Input: part model. Units: mm. Frame: model coordinates. Give positions to 0.01 mm unless a question says otherwise; leave off trailing zeros. Loops run counter-clockwise (first coordinate to the right, second up) from the corner with the lowest first, then second, coordinate; pieces in that order, holes last. Notation, with made-up numbers: (-23.75, -10.5) -> (-18.75, -10.5) arc R24 cw to (-18.75, 24.5) -> close; hole circle Ø6 at (15.5, -34.5). An arc over 180 degrees is marked (long way). Answer as a JSON object with one key per item and string values. Group by question number.
```python
from build123d import *

# Parameters (mm, degrees)
BASE_FLANGE1_DEPTH       = 2
SKETCH3_W                = 15
SKETCH3_H                = 15
TAB1_DEPTH               = 2
CUT_EXTRUDE1_REACH       = 314.176
SKETCH4_W                = 15
SKETCH4_H                = 45
M4_CLEARANCE_HOLE1_D     = 4.5
M4_CLEARANCE_HOLE1_DEPTH = 2
M3_CLEARANCE_HOLE1_D     = 3.2
CUT_EXTRUDE2_REACH       = 314.176
SKETCH10_W               = 24.5
SKETCH10_H               = 82
CUT_EXTRUDE3_REACH       = 314.176
SKETCH11_W               = 24.5
SKETCH11_H               = 165


# Sheet-metal steps are written as plain solids
with BuildPart() as part:
    # Sketch1 → Base-Flange1 (new body)
    with BuildSketch(Plane(origin=(0, 0, 0), x_dir=(1, 0, 0), z_dir=(0, 1, 0))):
        Polygon((-250, -150), (-235, -150), (-235, -165), (235, -165), (235, -150), (250, -150), (250, -135), (265, -135), (265, 135), (250, 135), (250, 150), (235, 150), (235, 165), (-235, 165), (-235, 150), (-250, 150), (-250, 135), (-265, 135), (-265, -135), (-250, -135), align=None)
    extrude(amount=-BASE_FLANGE1_DEPTH)

    # Sketch3 → Tab1 (add)
    with BuildSketch(Plane(origin=(0, 0, 0), x_dir=(1, 0, 0), z_dir=(0, 1, 0))):
        with Locations((-257.5, -142.5)):
            Rectangle(SKETCH3_W, SKETCH3_H)
    extrude(amount=-TAB1_DEPTH)

    # Sketch4 → Cut-Extrude1 (cut, up to next)
    with BuildSketch(Plane(origin=(0, 0, 0), x_dir=(1, 0, 0), z_dir=(0, 1, 0)), mode=Mode.PRIVATE) as cut_extrude1_sk1:
        with Locations((-257.5, -37.5)):
            Rectangle(SKETCH4_W, SKETCH4_H)
    cut_extrude1_tool1 = extrude(cut_extrude1_sk1.sketch, amount=-CUT_EXTRUDE1_REACH, mode=Mode.PRIVATE) & part.part
    add(cut_extrude1_tool1.solids().sort_by_distance((-257.5, 0, 37.5))[0], mode=Mode.SUBTRACT)

    # M4 Clearance Hole1
    with Locations(Plane(origin=(0, 0, 0), x_dir=(1, 0, 0), z_dir=(0, 1, 0))):
        with Locations((-260, -145), (-260, 0), (-260, 130), (-230, 160), (-80, 160), (80, 160), (230, 160), (260, 130), (260, 0), (260, -145), (230, -160), (80, -160), (-80, -160), (-230, -160)):
            Hole(M4_CLEARANCE_HOLE1_D / 2, depth=M4_CLEARANCE_HOLE1_DEPTH)

    # M3 Clearance Hole1 (through all)
    with Locations(Plane(origin=(0, 0, 0), x_dir=(1, 0, 0), z_dir=(0, 1, 0))):
        with Locations((221.5, -12.5), (171.5, -12.5), (171.5, 12.5), (221.5, 12.5), (75, 137.5), (5, 47.5), (75, 47.5), (5, 137.5), (-85, 52.5), (-110, -57.5), (-85, -57.5), (-110, 52.5), (-170, -57.5), (-195, 60.5), (-170, 60.5), (-195, -57.5), (25, 20), (50, -130), (25, -130), (50, 20)):
            Hole(M3_CLEARANCE_HOLE1_D / 2)

    # Sketch10 → Cut-Extrude2 (cut, up to next)
    with BuildSketch(Plane(origin=(0, 0, 0), x_dir=(1, 0, 0), z_dir=(0, 1, 0)), mode=Mode.PRIVATE) as cut_extrude2_sk1:
        with Locations((252.75, 84)):
            Rectangle(SKETCH10_W, SKETCH10_H)
    cut_extrude2_tool1 = extrude(cut_extrude2_sk1.sketch, amount=-CUT_EXTRUDE2_REACH, mode=Mode.PRIVATE) & part.part
    # Sketch10 → Cut-Extrude2 (cut, up to next)
    with BuildSketch(Plane(origin=(0, 0, 0), x_dir=(1, 0, 0), z_dir=(0, 1, 0)), mode=Mode.PRIVATE) as cut_extrude2_sk2:
        with Locations((252.75, -84)):
            Rectangle(SKETCH10_W, SKETCH10_H)
    cut_extrude2_tool2 = extrude(cut_extrude2_sk2.sketch, amount=-CUT_EXTRUDE2_REACH, mode=Mode.PRIVATE) & part.part
    add(cut_extrude2_tool1.solids().sort_by_distance((252.75, 0, -84))[0], mode=Mode.SUBTRACT)
    add(cut_extrude2_tool2.solids().sort_by_distance((252.75, 0, 84))[0], mode=Mode.SUBTRACT)

    # Sketch11 → Cut-Extrude3 (cut, up to next)
    with BuildSketch(Plane(origin=(0, 0, 0), x_dir=(1, 0, 0), z_dir=(0, 1, 0)), mode=Mode.PRIVATE) as cut_extrude3_sk1:
        with Locations((-252.75, 67.5)):
            Rectangle(SKETCH11_W, SKETCH11_H)
    cut_extrude3_tool1 = extrude(cut_extrude3_sk1.sketch, amount=-CUT_EXTRUDE3_REACH, mode=Mode.PRIVATE) & part.part
    add(cut_extrude3_tool1.solids().sort_by_distance((-252.75, 0, -67.5))[0], mode=Mode.SUBTRACT)


solid = part.part
```
Q1. Section C-C on z = 77. Return the cut outline in (x, y), then the cut area to 3 significant figures.
Q2. Pin query (flat end, axial travel): pin 1 Ø1 at (x, y) = (260, -0.5) entering from +Z; pin 2 Ø0.6 at (x, y) = (249.5, -1) entering from -Z. Return the tip coordinate at first contact, or that it passes through.
Q3. Section A-A on y = -1. State how many separate pieces and enclosed holes the cut face has, then the cut area to 3 significant figures.
Q4. Section B-B on z = -117.5. Return the cut outline in (x, y).
Q5. Ray query, probe 1 along Z at (x, y) = (5, -0.7); probe 2 along Z at (x, y) = (221.5, -0.8); probe 3 along X at (y, z) = (-1.05, -12.5). Return the intervals inside material, ascending.
Numbers:
{
 "1": {"outline": "(-265, -2) -> (240.5, -2) -> (240.5, 0) -> (-265, 0) -> close", "area": "1,010 mm²"},
 "2": {"pin 1": "stops at z = 135", "pin 2": "stops at z = -150"},
 "3": {"separate pieces": "1", "enclosed holes": "31", "area": "164,000 mm²"},
 "4": {"outline": "(-240.5, -2) -> (240.5, -2) -> (240.5, 0) -> (-240.5, 0) -> close"},
 "5": {"probe 1": "z = -165 to -139.1, -135.9 to -49.1, -45.9 to 165", "probe 2": "z = -165 to -14.1, -10.9 to 10.9, 14.1 to 165", "probe 3": "x = -240.5 to 169.9, 173.1 to 219.9, 223.1 to 265"}
}
